Geometry check sheet. Reference: drawing and pictorial views, mm from the part's lowest x, y, z. Round coordinates to 2 decimals unless told otherwise and drop trailing zeros. Write each loop counter-clockwise with the first axis right and the second up, starting at its lowest first coordinate (ties: lowest second). Pieces come first, ordered by that corner, then holes. Notation, with made-up numbers: M 33,-7 L 38,-7 A13 ccw 38,0 Z; hole C 40,84.25 d2. An arc over 180 degrees is marked long. Answer in a Markdown table with one row per item.
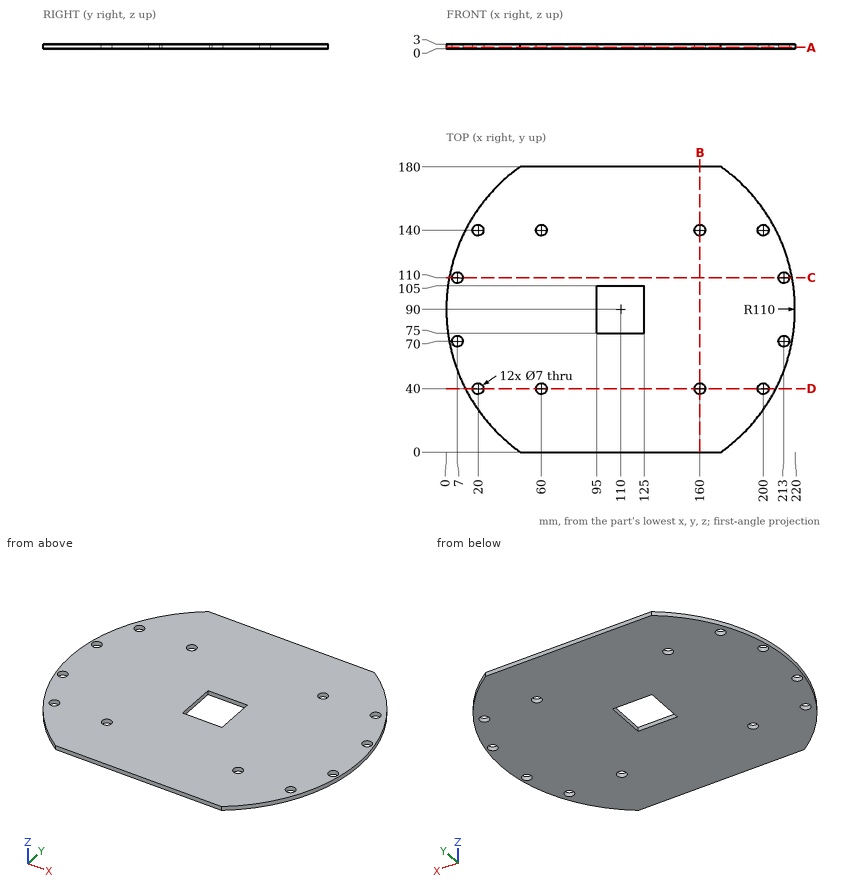
1. Go/stop test with a flat-tipped pin: pin 1 (1.5 mm diameter, centred on y = 89, z = 1, fed in from +X). Record where the tip stops, or that it passes through.
Found:
| item | result |
|---|---|
| pin 1 | stops at x = 220 |
2. Section check A-A, the plane z = 0.85. Count the separate pieces of the cut face and the enclosed holes in it, and give its area (3 significant figures).
Found:
| item | result |
|---|---|
| separate pieces | 1 |
| enclosed holes | 13 |
| area | 33,200 mm2 |
3. Section check D-D, the plane y = 40. Record the cut outline in (x, z).
Found:
| item | result |
|---|---|
| outline | M 12.02,0 L 16.5,0 L 16.5,3 L 12.02,3 Z; M 23.5,0 L 56.5,0 L 56.5,3 L 23.5,3 Z; M 63.5,0 L 156.5,0 L 156.5,3 L 63.5,3 Z; M 163.5,0 L 196.5,0 L 196.5,3 L 163.5,3 Z; M 203.5,0 L 207.98,0 L 207.98,3 L 203.5,3 Z |
4. Section check C-C, the plane y = 110. Record the cut outline in (x, z).
Found:
| item | result |
|---|---|
| outline | M 1.83,0 L 3.5,0 L 3.5,3 L 1.83,3 Z; M 10.5,0 L 209.5,0 L 209.5,3 L 10.5,3 Z; M 216.5,0 L 218.17,0 L 218.17,3 L 216.5,3 Z |
5. Section check B-B, the plane x = 160. Record the cut outline in (y, z), and give its area (3 significant figures).
Found:
| item | result |
|---|---|
| outline | M 0,0 L 36.5,0 L 36.5,3 L 0,3 Z; M 43.5,0 L 136.5,0 L 136.5,3 L 43.5,3 Z; M 143.5,0 L 180,0 L 180,3 L 143.5,3 Z |
| area | 498 mm2 |
6. Scan lines: L1, parallel to Y at x = 60, z = 1.5; L2, parallel to Y at x = 20, z = 2.3; L3, parallel to X at y = 137, z = 0.8. Record each from-to range of solid material in increasing order.
Found:
| item | result |
|---|---|
| L1 | y = 0 to 36.5, 43.5 to 136.5, 143.5 to 180 |
| L2 | y = 26.75 to 36.5, 43.5 to 136.5, 143.5 to 153.25 |
| L3 | x = 10.55 to 18.2, 21.8 to 58.2, 61.8 to 158.2, 161.8 to 198.2, 201.8 to 209.45 |
